Verification items for the finished model (mm, model axes). Face numbers are marked on the shaded views. A direction names the side the tool comes from. Coordinates: 2 decimals unless noted, no trailing zeros. Order: outer loops, then holes, each group sorted by start corner. A loop starts at its lowest first (then second) coordinate and runs counter-clockwise, first axis right, second up. Notation, with made-up numbers: (51, -24) -> (65, -24) arc R19 ccw to (65, -17) -> close; hole circle Ø8 at (-10.5, -8). An arc over 180 degrees is marked (long way). Answer as CSV lines item,"result".
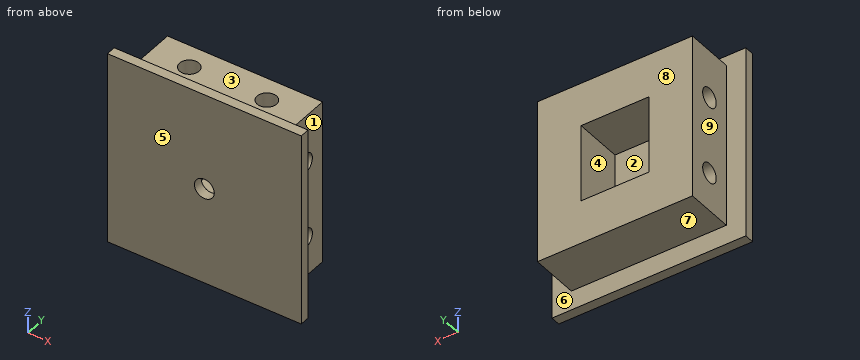
```python
from build123d import *

# Parameters (mm, degrees)
SKETCH003_W     = 40
SKETCH003_H     = 40
SKETCH003_R     = 2.05
PAD003_DEPTH    = 2
SKETCH006_W     = 32
SKETCH006_H     = 34
SKETCH006_W_2   = 14
SKETCH006_H_2   = 16
PAD005_DEPTH    = 10
SKETCH029_R     = 2
POCKET010_DEPTH = 8
SKETCH030_R     = 2
POCKET011_DEPTH = 8
SKETCH031_R     = 2
POCKET012_DEPTH = 8


with BuildPart() as part:
    # Sketch003 → Pad003 (new body)
    with BuildSketch(Plane.XZ):
        with Locations((0, 20)):
            Rectangle(SKETCH003_W, SKETCH003_H)
        with Locations((0, 20)):
            Circle(SKETCH003_R, mode=Mode.SUBTRACT)
    extrude(amount=PAD003_DEPTH)

    # Sketch006 (on Face6 of Pad003) → Pad005 (join)
    with BuildSketch(Plane(origin=(0, 0, 0), x_dir=(1, 0, 0), z_dir=(0, 1, 0))):
        with Locations((0, -21)):
            Rectangle(SKETCH006_W, SKETCH006_H)
        with Locations((0, -21)):
            Rectangle(SKETCH006_W_2, SKETCH006_H_2, mode=Mode.SUBTRACT)
    extrude(amount=PAD005_DEPTH)

    # Sketch029 (on Face8 of Pad005) → Pocket010 (cut)
    with BuildSketch(Plane(origin=(0, 0, 38), x_dir=(-1, 0, 0), z_dir=(0, 0, 1))):
        with Locations((-8, -5)):
            Circle(SKETCH029_R)
        with Locations((8, -5)):
            Circle(SKETCH029_R)
    extrude(amount=-POCKET010_DEPTH, mode=Mode.SUBTRACT)

    # Sketch030 (on Face7 of Pocket010) → Pocket011 (cut)
    with BuildSketch(Plane(origin=(-16, 0, 0), x_dir=(0, 0, -1), z_dir=(-1, 0, 0))):
        with Locations((-28, -5)):
            Circle(SKETCH030_R)
        with Locations((-12, -5)):
            Circle(SKETCH030_R)
    extrude(amount=-POCKET011_DEPTH, mode=Mode.SUBTRACT)

    # Sketch031 (on Face9 of Pocket011) → Pocket012 (cut)
    with BuildSketch(Plane(origin=(16, 0, 0), x_dir=(0, 0, 1), z_dir=(1, 0, 0))):
        with Locations((12, -5)):
            Circle(SKETCH031_R)
        with Locations((28, -5)):
            Circle(SKETCH031_R)
    extrude(amount=-POCKET012_DEPTH, mode=Mode.SUBTRACT)


with BuildPart() as part_1:
    # Body003 placement: moved
    add(part.part.moved(Location((0, -1000, 0))))


solid = part_1.part
```
Item 1: Section check B-B, the plane y = -999.5. Record the boundary of the cut face in (x, z), plus the area to 3 significant figures.
Answer list:
outline,"(-16, 4) -> (16, 4) -> (16, 38) -> (-16, 38) -> close; hole (-7, 13) -> (7, 13) -> (7, 29) -> (-7, 29) -> close"
area,"864 mm2"
Item 2: Tool access check on the marked faces 5, 6, 7, 8 and 9. Record the directions out of +Z, -Z, +X, -X, +Y, -Y that give a thin tool (end or side, any length) a straight path to the whole face; none if there is none.
Answer list:
face 5,"+Z, -Z, +X, -X, -Y"
face 6,"+Y"
face 7,"-Z, +X, -X, +Y"
face 8,"+Z, -Z, +X, -X, +Y"
face 9,"+Z, -Z, -X, +Y"
Item 3: Thickness scan on line 1 (Z direction, x = -10.5, y = -995); line 2 (Y direction, x = 12, z = 28); line 3 (Z direction, x = 2, y = -996.75). Record the ranges inside material, lowest first.
Answer list:
line 1,"4 to 10, 14 to 26, 30 to 38"
line 2,"-1002 to -997, -993 to -990"
line 3,"4 to 13, 29 to 38"
Item 4: Section check D-D, the plane x = -1. Record the boundary of the cut face in (y, z), plus the area to 3 significant figures.
Answer list:
outline,"(-1002, 0) -> (-1000, 0) -> (-1000, 4) -> (-990, 4) -> (-990, 13) -> (-1000, 13) -> (-1000, 18.21) -> (-1002, 18.21) -> close; (-1002, 21.79) -> (-1000, 21.79) -> (-1000, 29) -> (-990, 29) -> (-990, 38) -> (-1000, 38) -> (-1000, 40) -> (-1002, 40) -> close"
area,"253 mm2"
Item 5: Depth check by flat-ended pin: pin 1 Ø4.5 at (y, z) = (-995, 12) entering from +X; pin 2 Ø3 at (y, z) = (-995.5, 15) entering from -X; pin 3 Ø3 at (x, y) = (-8, -995) entering from +Z. Enter the tip coordinate at first touch or a pass-through.
Answer list:
pin 1,"x = 16"
pin 2,"x = -16"
pin 3,"z = 30"
Item 6: Section check A-A, the plane z = 20. Record the boundary of the cut face in (x, y).
Answer list:
outline,"(-20, -1002) -> (-2.05, -1002) -> (-2.05, -1000) -> (-7, -1000) -> (-7, -990) -> (-16, -990) -> (-16, -1000) -> (-20, -1000) -> close; (2.05, -1002) -> (20, -1002) -> (20, -1000) -> (16, -1000) -> (16, -990) -> (7, -990) -> (7, -1000) -> (2.05, -1000) -> close"
Item 7: Release check for a two-part mould opening along X. For the marked faces 1, 2, 3 and 4 record: +X half, -X half, draft (parallel to the pull), parting line (faces both ways), or undercut.
Answer list:
face 1,"+X half"
face 2,"undercut"
face 3,"draft"
face 4,"undercut"
Item 8: Section check C-C, the plane z = 34. Record the boundary of the cut face in (x, y).
Answer list:
outline,"(-20, -1002) -> (20, -1002) -> (20, -1000) -> (16, -1000) -> (16, -990) -> (-16, -990) -> (-16, -1000) -> (-20, -1000) -> close; hole circle Ø4 at (-8, -995); hole circle Ø4 at (8, -995)"
